```python
from build123d import *

# Parameters (mm, degrees)
BOSS_EXTRUDE1_DEPTH = 4.6
CUT_EXTRUDE1_DEPTH  = 164.683291756
FILLET1_R           = 0.5


with BuildPart() as part:
    # Sketch1 → Boss-Extrude1 (new body)
    with BuildSketch(Plane.XY):
        Polygon((8.2, 146), (8.2, 155.5), (18.2, 155.5), (18.2, 146), (28.2, 146), (28.2, 155.5), (38.2, 155.5), (38.2, 146), (46.4, 146), (46.4, 123), (50.9, 123), (50.9, 103), (46.4, 103), (46.4, 83), (50.9, 83), (50.9, 63), (46.4, 63), (46.4, 43), (50.9, 43), (50.9, 23), (46.4, 23), (46.4, 0), (30.7, 0), (30.7, -14.5), (15.7, -14.5), (15.7, 0), (0, 0), (0, 146), align=None)
    extrude(amount=BOSS_EXTRUDE1_DEPTH)

    # Sketch2 → Cut-Extrude1 (cut, through all)
    with BuildSketch(Plane.XY.offset(4.6)):
        with BuildLine():
            Line((15.7, 0), (15.7, -5))
            ThreePointArc((15.7, -5), (14.2, -6.5), (12.7, -5))
            Line((12.7, -5), (12.7, 0))
            ThreePointArc((12.7, 0), (14.2, 1.5), (15.7, 0))
        make_face()
        with BuildLine():
            Line((30.7, 0), (30.7, -5))
            ThreePointArc((30.7, -5), (32.2, -6.5), (33.7, -5))
            Line((33.7, -5), (33.7, 0))
            ThreePointArc((33.7, 0), (32.2, 1.5), (30.7, 0))
        make_face()
        with BuildLine():
            Line((46.4, 23), (50.9, 23))
            ThreePointArc((50.9, 23), (52.4, 21.5), (50.9, 20))
            Line((50.9, 20), (46.4, 20))
            ThreePointArc((46.4, 20), (44.9, 21.5), (46.4, 23))
        make_face()
        with BuildLine():
            Line((46.4, 63), (50.9, 63))
            ThreePointArc((50.9, 63), (52.4, 61.5), (50.9, 60))
            Line((50.9, 60), (46.4, 60))
            ThreePointArc((46.4, 60), (44.9, 61.5), (46.4, 63))
        make_face()
        with BuildLine():
            Line((46.4, 103), (50.9, 103))
            ThreePointArc((50.9, 103), (52.4, 101.5), (50.9, 100))
            Line((50.9, 100), (46.4, 100))
            ThreePointArc((46.4, 100), (44.9, 101.5), (46.4, 103))
        make_face()
        with BuildLine():
            Line((46.4, 43), (50.9, 43))
            ThreePointArc((50.9, 43), (52.4, 44.5), (50.9, 46))
            Line((50.9, 46), (46.4, 46))
            ThreePointArc((46.4, 46), (44.9, 44.5), (46.4, 43))
        make_face()
        with BuildLine():
            Line((46.4, 83), (50.9, 83))
            ThreePointArc((50.9, 83), (52.4, 84.5), (50.9, 86))
            Line((50.9, 86), (46.4, 86))
            ThreePointArc((46.4, 86), (44.9, 84.5), (46.4, 83))
        make_face()
        with BuildLine():
            Line((46.4, 123), (50.9, 123))
            ThreePointArc((50.9, 123), (52.4, 124.5), (50.9, 126))
            Line((50.9, 126), (46.4, 126))
            ThreePointArc((46.4, 126), (44.9, 124.5), (46.4, 123))
        make_face()
        with BuildLine():
            Line((38.2, 146), (38.2, 155.5))
            ThreePointArc((38.2, 155.5), (39.7, 157), (41.2, 155.5))
            Line((41.2, 155.5), (41.2, 146))
            ThreePointArc((41.2, 146), (39.7, 144.5), (38.2, 146))
        make_face()
        with BuildLine():
            Line((28.2, 146), (28.2, 155.5))
            ThreePointArc((28.2, 155.5), (26.7, 157), (25.2, 155.5))
            Line((25.2, 155.5), (25.2, 146))
            ThreePointArc((25.2, 146), (26.7, 144.5), (28.2, 146))
        make_face()
        with BuildLine():
            Line((8.2, 146), (8.2, 155.5))
            ThreePointArc((8.2, 155.5), (6.7, 157), (5.2, 155.5))
            Line((5.2, 155.5), (5.2, 146))
            ThreePointArc((5.2, 146), (6.7, 144.5), (8.2, 146))
        make_face()
        with BuildLine():
            Line((18.2, 146), (18.2, 155.5))
            ThreePointArc((18.2, 155.5), (19.7, 157), (21.2, 155.5))
            Line((21.2, 155.5), (21.2, 146))
            ThreePointArc((21.2, 146), (19.7, 144.5), (18.2, 146))
        make_face()
    extrude(amount=-CUT_EXTRUDE1_DEPTH, mode=Mode.SUBTRACT)

    # Fillet1
    fillet1_edges = [part.edges().sort_by_distance(p)[0] for p in [
        (0, 146, 2.3),
        (8.2, 155.5, 2.3),
        (18.2, 155.5, 2.3),
        (28.2, 155.5, 2.3),
        (38.2, 155.5, 2.3),
        (46.4, 146, 2.3),
        (50.9, 123, 2.3),
        (50.9, 103, 2.3),
        (50.9, 83, 2.3),
        (50.9, 63, 2.3),
        (50.9, 43, 2.3),
        (50.9, 23, 2.3),
        (46.4, 0, 2.3),
        (30.7, -14.5, 2.3),
        (15.7, -14.5, 2.3),
        (0, 0, 2.3),
    ]]
    fillet(fillet1_edges, radius=FILLET1_R)


solid = part.part
```
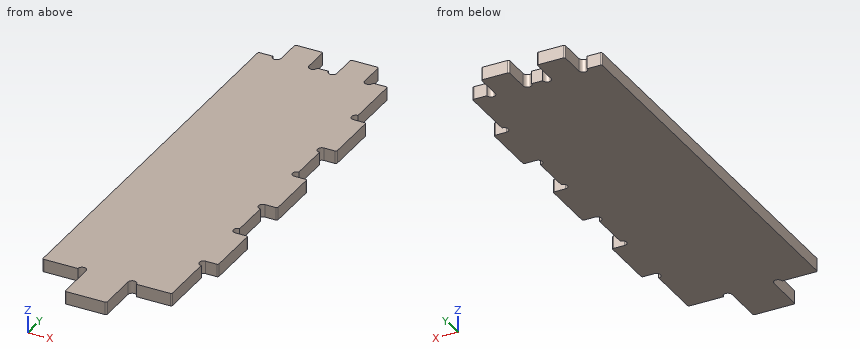
Input: part model. Units: mm. Frame: model coordinates. Give positions to 0.01 mm unless a question says otherwise; leave off trailing zeros. Order: outer loops, then holes, each group sorted by start corner. A loop starts at its lowest first (then second) coordinate and runs counter-clockwise, first axis right, second up. Notation, with made-up numbers: (79.5, 28.5) - (109.5, 28.5) arc R21 ccw to (109.5, 43.5) - close; hole circle Ø5 at (-20, 67.5). An arc over 180 degrees is marked (long way). Use a Markdown table: item, result.
(1) Section query B-B (y = 101.5). Output: boundary loops of the cut face in (x, z), then the cut area to 3 significant figures.
Computed values:
| item | result |
|---|---|
| outline | (0, 0) - (44.9, 0) - (44.9, 4.6) - (0, 4.6) - close |
| area | 207 mm2 |
(2) Line query: line 1 (Y direction, x = 48.5, z = 0.4); line 2 (X direction, y = 48, z = 4.3); line 3 (Y direction, x = 35.5, z = 2). Output: solid intervals per line, ascending. Write a range as from..to.
Computed values:
| item | result |
|---|---|
| line 1 | y = 23..43, 63..83, 103..123 |
| line 2 | x = 0..46.4 |
| line 3 | y = 0..155.5 |
(3) Pin query (flat end, axial travel): pin 1 (3 mm diameter, centred on x = 30, y = 116.5, fed in from -Z); pin 2 (2.5 mm diameter, centred on y = -8, z = 1.5, fed in from -X); pin 3 (2 mm diameter, centred on x = 47.5, z = 3, fed in from +Y); pin 4 (2 mm diameter, centred on x = 23, z = 1.5, fed in from +Y). Return the tip coordinate at first contact, or that it passes through.
Computed values:
| item | result |
|---|---|
| pin 1 | stops at z = 0 |
| pin 2 | stops at x = 15.7 |
| pin 3 | stops at y = 123 |
| pin 4 | stops at y = 146 |
(4) Section query A-A (x = 6.7). Output: boundary loops of the cut face in (y, z), then the cut area to 3 significant figures.
Computed values:
| item | result |
|---|---|
| outline | (0, 0) - (144.5, 0) - (144.5, 4.6) - (0, 4.6) - close |
| area | 665 mm2 |
